Could you check a few things on this drawing? It's one solid part, dimensions in mm from its lowest x, y, z. Round coordinates to 2 decimals unless told otherwise and drop trailing zeros. Write each loop counter-clockwise with the first axis right and the second up, starting at its lowest first coordinate (ties: lowest second). Pieces come first, ordered by that corner, then holes. Notation, with made-up numbers: M 18,32 L 42,32 A14 cw 42,49 Z; hole C -13.5,1.25 d7. An arc over 180 degrees is marked long. One line per item, written item: value. Start each with the question number.
(1) I want a section at A-A on x = 81.5. Please give me the cut outline in (y, z).
(2) I'm going to push flat-ended pins straight in: pin 1 Ø1.5 at (x, y) = (113.5, 2) entering from +Z; pin 2 Ø2 at (x, z) = (51.5, 44.5) entering from -Y; pin 3 Ø7 at (x, z) = (81.5, 30) entering from -Y; pin 4 Ø0.9 at (x, y) = (116, 2) entering from +Z. Where does each tip first touch, or does it pass through?
(3) I want a section at B-B on y = 1.7. Count the separate pieces of the cut face and the enclosed holes in it, and give its area (3 significant figures).
(4) If I drill on L1, parallel to Z at x = 88.5, y = 2.65; L2, parallel to X at y = 1.4, z = 6.5; L3, parallel to Z at x = 71, y = 0.45, over which ranges is the centre line in solid material (lowest first)?
(5) I want a section at D-D on z = 5. Please give me the cut outline in (x, y).
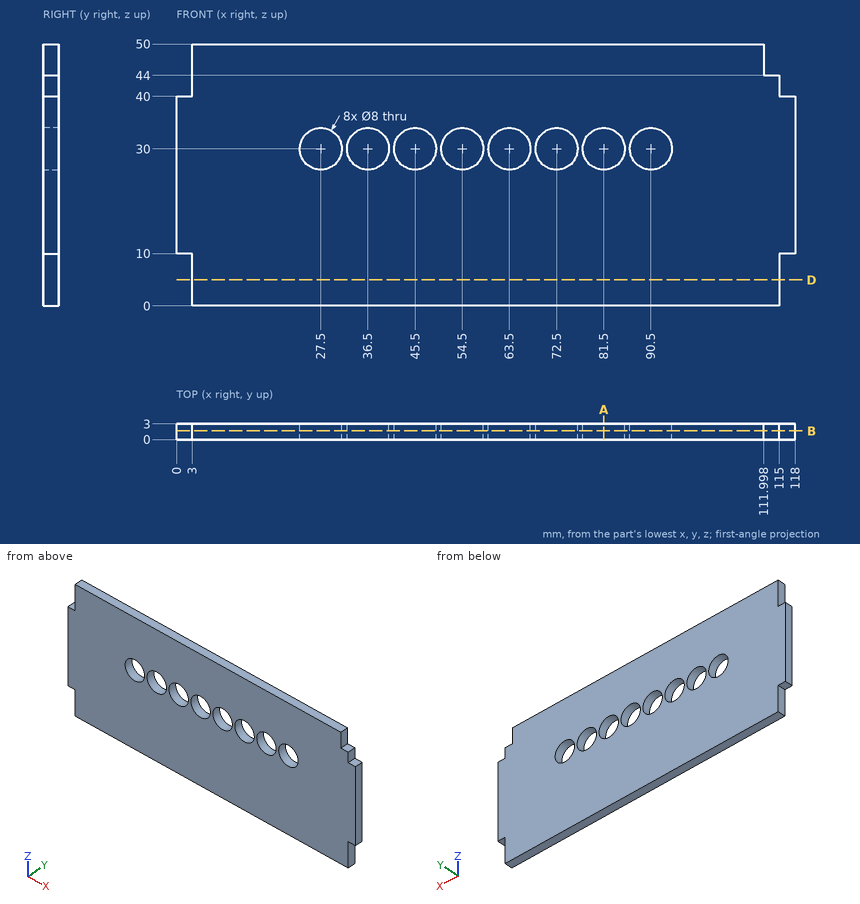
Found:
1. outline: M 0,0 L 3,0 L 3,26 L 0,26 Z; M 0,34 L 3,34 L 3,50 L 0,50 Z
2. pin 1: stops at z = 44
2. pin 2: stops at y = 0
2. pin 3: passes through
2. pin 4: stops at z = 40
3. separate pieces: 1
3. enclosed holes: 8
3. area: 5,360 mm²
4. L1: z = 0 to 26.54, 33.46 to 50
4. L2: x = 3 to 115
4. L3: z = 0 to 26.29, 33.71 to 50
5. outline: M 3,0 L 115,0 L 115,3 L 3,3 Z
